The listing builds one solid part. Answer for the finished solid, in the listing's coordinates (mm). A direction names the side the tool comes from. Coordinates: 2 decimals unless noted, no trailing zeros. Order: outer loops, then holes, each group sorted by start corner. A loop starts at its lowest first (then second) coordinate and runs counter-clockwise, first axis right, second up.
```python
from build123d import *

# Parameters (mm, degrees)
SKETCH1_R                    = 16.5
BOSS_EXTRUDE1_DEPTH          = 5
CHAMFER2_SIZE                = 1
CHAMFER2_SIZE2               = 5
SKETCH3_R                    = 13.5
CUT_EXTRUDE1_DEPTH           = 2.78
SKETCH5_W                    = 1
SKETCH5_H                    = 2
REVOLVE4_ANGLE               = 5
REVOLVE4_OTHER_WAY_ANGLE     = 5
REVOLVE6_DEPTH               = 2
SKETCH9_W                    = 16.5
SKETCH9_H                    = 2
CUT_REVOLVE1_ANGLE           = 85
CUT_REVOLVE1_OTHER_WAY_ANGLE = 10


# Read off the part's stored shape, not the designer's step: Revolve6
with BuildPart() as part:
    # Sketch1 → Boss-Extrude1 (new body)
    with BuildSketch(Plane(origin=(0, 0, 0), x_dir=(1, 0, 0), z_dir=(0, 1, 0))):
        with Locations(Location((0, 0, 0), (0, 0, 270))):
            Circle(SKETCH1_R)
    extrude(amount=BOSS_EXTRUDE1_DEPTH)

    # Chamfer2
    chamfer2_edges = [part.edges().sort_by_distance(p)[0] for p in [
        (0, 5, -16.5),
    ]]
    chamfer2_side = [part.faces().sort_by_distance(p)[0] for p in [
        (0, 2.5, -16.5),
    ]]
    chamfer(chamfer2_edges, length=CHAMFER2_SIZE, length2=CHAMFER2_SIZE2, reference=chamfer2_side[0])

    # Sketch3 → Cut-Extrude1 (cut)
    with BuildSketch(Plane(origin=(0, 0, 0), x_dir=(1, 0, 0), z_dir=(0, 1, 0))):
        with Locations(Location((0, 0, 0), (0, 0, 270))):
            Circle(SKETCH3_R)
    extrude(amount=CUT_EXTRUDE1_DEPTH, mode=Mode.SUBTRACT)

    # Sketch5 → Revolve4 (revolve)
    with BuildSketch(Plane(origin=(0, 0, 0), x_dir=(0, 0, -1), z_dir=(1, 0, 0))):
        with Locations((17, 1)):
            Rectangle(SKETCH5_W, SKETCH5_H)
    revolve(axis=Axis((0, 0, 0), (0, 1, 0)), revolution_arc=REVOLVE4_ANGLE)

    # Sketch5 → Revolve4 other way (revolve)
    with BuildSketch(Plane(origin=(0, 0, 0), x_dir=(0, 0, -1), z_dir=(1, 0, 0))):
        with Locations((17, 1)):
            Rectangle(SKETCH5_W, SKETCH5_H)
    revolve(axis=Axis((0, 0, 0), (0, -1, 0)), revolution_arc=REVOLVE4_OTHER_WAY_ANGLE)

    # Revolve6 outline → Revolve6 (add)
    with BuildSketch(Plane(origin=(0, 0, 0), x_dir=(1, 0, 0), z_dir=(0, 1, 0))):
        with BuildLine():
            ThreePointArc((-1.525225498, -17.433407217), (0, -17.5), (1.525225498, -17.433407217))
            Line((1.525225498, -17.433407217), (1.438069755, -16.437212519))
            ThreePointArc((1.438069755, -16.437212519), (0, -16.5), (-1.438069755, -16.437212519))
            Line((-1.438069755, -16.437212519), (-1.525225498, -17.433407217))
        make_face()
    extrude(amount=REVOLVE6_DEPTH)

    # Sketch9 → Cut-Revolve1 (revolve, cut)
    with BuildSketch(Plane.XY):
        with Locations((-8.25, 1)):
            Rectangle(SKETCH9_W, SKETCH9_H)
    revolve(axis=Axis((0, 0, 0), (0, 1, 0)), revolution_arc=CUT_REVOLVE1_ANGLE, mode=Mode.SUBTRACT)

    # Sketch9 → Cut-Revolve1 other way (revolve, cut)
    with BuildSketch(Plane.XY):
        with Locations((-8.25, 1)):
            Rectangle(SKETCH9_W, SKETCH9_H)
    revolve(axis=Axis((0, 0, 0), (0, -1, 0)), revolution_arc=CUT_REVOLVE1_OTHER_WAY_ANGLE, mode=Mode.SUBTRACT)


solid = part.part
```
1) The mould has two halves that part along Z. Classify faces 1 (the flat face through (12, 0, -7)), 2 (the conical face through (-11.46, 4.95, -2.55)), 3 (the flat face through (-1.48, 1.01, -16.93)), 4 (the cylindrical face through (9.124, 1.371, -9.95)): released by +Z, released by -Z, zero draft, split by the parting line, or undercut.
2) Straight lines are drawn through the part: probe 1 along Z at (x, y) = (0, 2.1); probe 2 along X at (y, z) = (1.3, 0); probe 3 along Y at (x, z) = (5.5, -9). For each, find the intervals that lie inside material, in ascending order.
3) For faces 5 (the flat face through (1.482, 0.986, 16.942)), 6 (the flat face through (-14.793, 1.014, -2.608)), 7 (the flat face through (0, 2.78, 0)), 8 (the cylindrical face through (0, 1, 17.5)), 9 (the flat face through (0, 5, 0)), determine the directions among +Z, -Z, +X, -X, +Y, -Y from which every point of the face is accessible in a straight line to the end or side of a thin tool.
4) A cutting plane is placed at B-B, the plane x = 0. Write down the section's boundary in (y, z).
5) A cutting plane is placed at A-A, the plane z = 0. Write down the section's boundary in (x, y), plus the area to 3 significant figures.
6) Each of these flat-tipped pins is pushed along its axis until it touches: P1, Ø2, axis at x = -8.5, y = 3, coming from the +Z side; P2, Ø1.5, axis at x = -1, y = 4, coming from the +Z side; P3, Ø1, axis at y = 3.5, z = -13.5, coming from the +X side. Where does it stop, or does it pass through?
Working result:
1. face 1: zero draft
1. face 2: split by the parting line
1. face 3: undercut
1. face 4: undercut
2. probe 1: z = -16.5 to -13.5, 13.5 to 16.5
2. probe 2: x = 13.5 to 16.5
2. probe 3: y = 2.78 to 5
3. face 5: +X, +Y, -Y
3. face 6: +Z, -X, -Y
3. face 7: -Y
3. face 8: +Z, +Y, -Y
3. face 9: +Z, -Z, +X, -X, +Y
4. outline: (0, -17.5) - (2, -17.5) - (2, -16.5) - (4, -16.5) - (5, -11.5) - (5, 11.5) - (4, 16.5) - (2, 16.5) - (2, 17.5) - (0, 17.5) - (0, 13.5) - (2.78, 13.5) - (2.78, -13.5) - (0, -13.5) - close
5. outline: (-16.5, 2) - (-13.5, 2) - (-13.5, 2.78) - (13.5, 2.78) - (13.5, 0) - (16.5, 0) - (16.5, 4) - (11.5, 5) - (-11.5, 5) - (-16.5, 4) - close
5. area: 78.9 mm2
6. P1: stops at z = 14.7
6. P2: stops at z = 16.5
6. P3: stops at x = 10.16
